```python
from build123d import *

# Parameters (mm, degrees)
F0_R     = 5
F1_DEPTH = 50
F2_R     = 3


with BuildPart() as f1:
    # F0 (on Top) → F1 (new body)
    with BuildSketch(Plane.XY):
        Circle(F0_R)
    extrude(amount=F1_DEPTH)

    # F4: sweep along a path in F3
    with BuildLine(Plane.XZ) as f4_path:
        Line((0, 50), (0, 70.065357))
        ThreePointArc((0, 70.065357), (-2.906012, 77.11343), (-9.935066, 80.065146))
        Line((-9.935066, 80.065146), (-50, 80.325309))
    # F2 (on face) → F4 (sweep)
    with BuildSketch(Plane.XY.offset(50)):
        Circle(F2_R)
    sweep(path=f4_path.line)


solid = f1.part
```
Geometry: final body of the model. Coordinates: model frame, mm. Coordinates: 2 decimals unless noted, no trailing zeros. Write each loop counter-clockwise with the first axis right and the second up, starting at its lowest first coordinate (ties: lowest second). Pieces come first, ordered by that corner, then holes. Notation, with made-up numbers: M -38,50 L -18,50 A19 cw -18,58 Z; hole C 65.5,11 d2. An arc over 180 degrees is marked long. Answer as CSV lines item,"result". Start each with the question number.
Q1. Cut plane B-B on z = 17. Return the cut outline in (x, y).
Q2. Line query: line 1 (Z direction, x = -4, y = -1); line 2 (Z direction, x = 3.5, y = 0); line 3 (X direction, y = -3.75, z = 16). Output: solid intervals per line, ascending. Write a range as from..to.
Q3. Cut plane A-A on z = 60.5. Return the cut outline in (x, y), then the cut area to 3 significant figures.
Q4. Pin query (flat end, axial travel): P1, Ø5, axis at x = -30.5, y = -0.5, coming from the +Z side; P2, Ø3, axis at x = 2, y = -2.5, coming from the +Z side; P3, Ø1.5, axis at x = -2.5, y = -1.5, coming from the +Z side. Return the tip coordinate at first contact, or that it passes through.
Q5. Mould query, pull axis Z, two halves, no side actions, for faces 1 (the flat face through (0, 0, 0)), 2 (the cylindrical face through (-1.08, -4.88, 24.65)), 3 (the flat face through (-0.1, -3.3, 50)). Classes: released by +Z, released by -Z, zero draft, split by the parting line, or undercut.
Findings below:
1,outline,"C 0,0 d10"
2,line 1,"z = 0..50, 73.99..81.4"
2,line 2,"z = 0..50"
2,line 3,"x = -3.31..3.31"
3,outline,"C 0,0 d6"
3,area,"28.3 mm2"
4,P1,"stops at z = 83.21"
4,P2,"stops at z = 76.43"
4,P3,"stops at z = 80.86"
5,face 1,"released by -Z"
5,face 2,"zero draft"
5,face 3,"undercut"
